Source: CAD feature listing. Evaluate the final solid. Frame: model axes, mm. Round coordinates to 2 decimals unless told otherwise and drop trailing zeros. Loops run counter-clockwise (first coordinate to the right, second up) from the corner with the lowest first, then second, coordinate; pieces in that order, holes last.
(1) Section C-C, the plane y = 42. Return the cut outline in (x, z).
(2) First-contact query: pin 1 Ø1.4 at (x, z) = (2, 0) entering from -Y; pin 2 Ø1.8 at (x, y) = (0, 42.88) entering from +Z (3 decimals); pin 3 Ø12 at (x, y) = (-2, 37) entering from +Z; pin 4 Ø1.4 at (x, z) = (5, 0) entering from +Y. Flat tips, straight axial feed; report the tip coordinate or a pass-through.
(3) Material intervals for probe 1 along Y at (x, z) = (1.25, -0.9); probe 2 along Y at (x, z) = (0, 0); probe 3 along Y at (x, z) = (-4, 1.35), sorted ascending.
(4) Section A-A, the plane y = 0. Return the cut outline in (x, z), plus the area to 3 significant figures.
(5) Section B-B, the plane z = -0.75. Return the cut outline in (x, y).
```python
from build123d import *

# Parameters (mm, degrees)
SKETCH_1_R          = 0.75
SKETCH_1_W          = 13
SKETCH_1_H          = 23
SKETCH_1_R_2        = 1.5
EXTRUDE_1_DEPTH     = 1.45
SKETCH_2_W          = 6
SKETCH_2_H          = 1
CUT_EXTRUDE_1_DEPTH = 3
FILLET_1_R          = 0.3


with BuildPart() as part:
    # 草图1 → 凸台-拉伸1 (new body, symmetric)
    with BuildSketch(Plane.XY):
        with BuildLine():
            ThreePointArc((-10, -8), (0, -18), (10, -8))
            Line((10, -8), (10, 6))
            Line((10, 6), (4.955472685, 43.54580062))
            ThreePointArc((4.955472685, 43.54580062), (-2.725773115, 47.071677579), (-2.618575221, 38.62053245))
            ThreePointArc((-2.618575221, 38.62053245), (-0.423906888, 35.714832413), (-0.782117822, 32.091112401))
            Line((-0.782117822, 32.091112401), (-10, 14))
            Line((-10, 14), (-10, -8))
        make_face()
        with Locations((0, -13.7)):
            Circle(SKETCH_1_R, mode=Mode.SUBTRACT)
        Rectangle(SKETCH_1_W, SKETCH_1_H, mode=Mode.SUBTRACT)
        with Locations((0, 13.7)):
            Circle(SKETCH_1_R, mode=Mode.SUBTRACT)
        with Locations((0, 42.88)):
            Circle(SKETCH_1_R_2, mode=Mode.SUBTRACT)
        Polygon((5.562298916, 16.5), (-5.359207663, 16.5), (3.283346167, 33.461966942), align=None, mode=Mode.SUBTRACT)
    extrude(amount=EXTRUDE_1_DEPTH, both=True)

    # 草图2 → 切除-拉伸1 (cut)
    with BuildSketch(Plane.XY.offset(1.45)):
        with Locations((0, -12)):
            Rectangle(SKETCH_2_W, SKETCH_2_H)
    extrude(amount=-CUT_EXTRUDE_1_DEPTH, mode=Mode.SUBTRACT)

    # 圆角1
    fillet_1_edges = [part.edges().sort_by_distance(p)[0] for p in [
        (-3, -11.5, 0),
        (3, -11.5, 0),
        (3, -12.5, 0),
        (-3, -12.5, 0),
    ]]
    fillet(fillet_1_edges, radius=FILLET_1_R)


solid = part.part
```
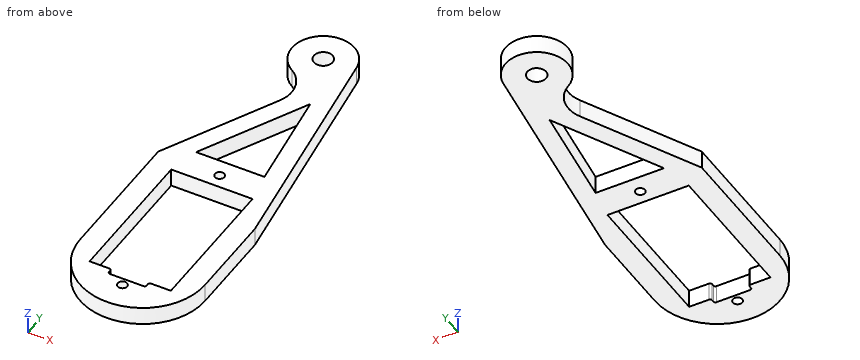
Output values:
1. outline: (-4.92, -1.45) - (-1.21, -1.45) - (-1.21, 1.45) - (-4.92, 1.45) - close; (1.21, -1.45) - (5.16, -1.45) - (5.16, 1.45) - (1.21, 1.45) - close
2. pin 1: stops at y = -17.92
2. pin 2: passes through
2. pin 3: stops at z = 1.45
2. pin 4: stops at y = 45.43
3. probe 1: y = -17.92 to -12.5, 11.5 to 16.5, 29.47 to 42.05, 43.71 to 47.72
3. probe 2: y = -18 to -14.45, -12.95 to -12.5, 11.5 to 12.95, 14.45 to 16.5, 27.02 to 41.38, 44.38 to 47.88
3. probe 3: y = -17.17 to -11.5, 11.5 to 16.5, 19.17 to 25.78, 39.88 to 45.88
4. outline: (-10, -1.45) - (-6.5, -1.45) - (-6.5, 1.45) - (-10, 1.45) - close; (6.5, -1.45) - (10, -1.45) - (10, 1.45) - (6.5, 1.45) - close
4. area: 20.3 mm2
5. outline: (-10, -8) arc R10 ccw to (10, -8) - (10, 6) - (4.96, 43.55) arc R5 ccw (long way) to (-2.62, 38.62) arc R5 cw to (-0.78, 32.09) - (-10, 14) - close; hole (-6.5, -11.5) - (-3.3, -11.5) arc R0.3 cw to (-3, -11.8) - (-3, -12.2) arc R0.3 ccw to (-2.7, -12.5) - (2.7, -12.5) arc R0.3 ccw to (3, -12.2) - (3, -11.8) arc R0.3 cw to (3.3, -11.5) - (6.5, -11.5) - (6.5, 11.5) - (-6.5, 11.5) - close; hole (-5.36, 16.5) - (5.56, 16.5) - (3.28, 33.46) - close; hole circle Ø3 at (0, 42.88); hole circle Ø1.5 at (0, -13.7); hole circle Ø1.5 at (0, 13.7)
